Source: CAD feature listing. Evaluate the final solid. Frame: model axes, mm. Round coordinates to 2 decimals unless told otherwise and drop trailing zeros. Loops run counter-clockwise (first coordinate to the right, second up) from the corner with the lowest first, then second, coordinate; pieces in that order, holes last. Notation, with made-up numbers: M 22,-24 L 58,-24 A25 ccw 58,-7 Z; hole C -5,52 d7. An arc over 180 degrees is marked long. One line per item, written item: value.
Autodesk Inventor part; units mm, degrees
ref_plane "YZ Plane" through (0, 0, 0) normal (1, 0, 0) x (0, 1, 0)
ref_plane "XZ Plane" through (0, 0, 0) normal (0, 1, 0) x (-1, 0, 0)
ref_plane "XY Plane" through (0, 0, 0) normal (0, 0, 1) x (1, 0, 0)
sketch "スケッチ1" plane through (0, 0, 0) normal (0, 0, 1) x (1, 0, 0)
  circle A0 centre (0, 0) radius 1
  dimension "d0" = 2
extrude "押し出し1" add sketch "スケッチ1" along normal blind 4
sketch "スケッチ2" plane through (0, 0, 4) normal (0, 0, 1) x (1, 0, 0)
  circle A0 centre (0, 0) radius 1
  circle A1 centre (0, 0) radius 2
  dimension "d3" = 4
extrude "押し出し2" add sketch "スケッチ2" along normal blind 1.5 contours A0 | A1
chamfer "面取り1" distance 1 angle 45 1 edges at (-2, 0, 4)
thread "ねじ1"
sketch "スケッチ3" plane through (0, 0, 0) normal (0, 0, -1) x (-1, 0, 0)
  circle A0 centre (0, 0) radius 1
extrude "押し出し3" add sketch "スケッチ3" along normal blind 0.5
properties part number "SB M2 8mm皿ネジ" material "Steel"
1. Section query C-C (z = 1.9). Return the cut outline in (x, y), and give its area (3 significant figures).
Report:
outline: C 0,0 d2
area: 3.14 mm2
2. Pin query (flat end, axial travel): pin 1 (1.5 mm diameter, centred on x = 0.5, z = 2.5, fed in from -Y). Return the tip coordinate at first contact, or that it passes through.
Report:
pin 1: stops at y = -1
3. Ray query, line 1 (X direction, y = 0, z = 1.15); line 2 (Z direction, x = -0.5, y = 0.9); line 3 (Y direction, x = 0.8, z = 3.35). Return the intervals inside material, ascending. Write a range as [from, to].
Report:
line 1: x = [-1, 1]
line 2: z = [4.03, 5.5]
line 3: y = [-0.6, 0.6]
